Check sheet for the modelled part. Datum: model origin and axes. Units: mm. Coordinates: 2 decimals unless noted, no trailing zeros. Loops run counter-clockwise (first coordinate to the right, second up) from the corner with the lowest first, then second, coordinate; pieces in that order, holes last.
```python
from build123d import *

# Parameters (mm, degrees)
BOSS_EXTRUDE1_DEPTH = 2.5
FILLET1_R           = 3
FILLET2_R           = 3
FILLET4_R           = 3
FILLET5_R           = 3
SKETCH2_R           = 3
CUT_EXTRUDE1_DEPTH  = 3
FILLET6_R           = 3
FILLET7_R           = 3


with BuildPart() as part:
    # Sketch1 → Boss-Extrude1 (new body)
    with BuildSketch(Plane(origin=(0, 0, 0), x_dir=(1, 0, 0), z_dir=(0, 1, 0))):
        Polygon((-12.469879518, 24.84939759), (17.530120482, 24.84939759), (17.530120482, -5.15060241), (47.530120482, -5.15060241), (47.530120482, -35.15060241), (17.530120482, -35.15060241), (-12.469879518, -35.15060241), (-42.469879518, -35.15060241), (-42.469879518, -5.15060241), (-12.469879518, -5.15060241), align=None)
    extrude(amount=BOSS_EXTRUDE1_DEPTH)

    # Fillet1
    fillet1_edges = [part.edges().sort_by_distance(p)[0] for p in [
        (-42.469879518, 1.25, 5.15060241),
    ]]
    fillet(fillet1_edges, radius=FILLET1_R)

    # Fillet2
    fillet2_edges = [part.edges().sort_by_distance(p)[0] for p in [
        (-42.469879518, 1.25, 35.15060241),
    ]]
    fillet(fillet2_edges, radius=FILLET2_R)

    # Fillet4
    fillet4_edges = [part.edges().sort_by_distance(p)[0] for p in [
        (17.530120482, 1.25, -24.84939759),
    ]]
    fillet(fillet4_edges, radius=FILLET4_R)

    # Fillet5
    fillet5_edges = [part.edges().sort_by_distance(p)[0] for p in [
        (-12.469879518, 1.25, -24.84939759),
    ]]
    fillet(fillet5_edges, radius=FILLET5_R)

    # Sketch2 → Cut-Extrude1 (cut)
    with BuildSketch(Plane(origin=(0, 2.5, 0), x_dir=(1, 0, 0), z_dir=(0, 1, 0))):
        with Locations((2.530120482, 9.84939759)):
            Circle(SKETCH2_R)
        with Locations((-27.469879518, -20.15060241)):
            Circle(SKETCH2_R)
        with Locations((32.530120482, -20.15060241)):
            Circle(SKETCH2_R)
    extrude(amount=-CUT_EXTRUDE1_DEPTH, mode=Mode.SUBTRACT)

    # Fillet6
    fillet6_edges = [part.edges().sort_by_distance(p)[0] for p in [
        (47.530120482, 1.25, 35.15060241),
    ]]
    fillet(fillet6_edges, radius=FILLET6_R)

    # Fillet7
    fillet7_edges = [part.edges().sort_by_distance(p)[0] for p in [
        (47.530120482, 1.25, 5.15060241),
    ]]
    fillet(fillet7_edges, radius=FILLET7_R)


solid = part.part
```
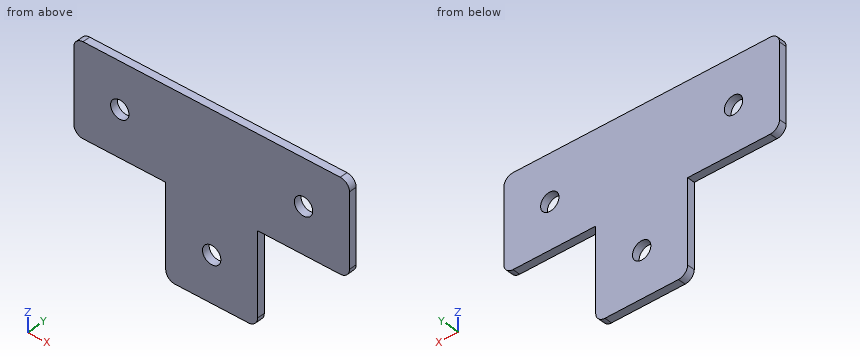
1) Section check D-D on z = -2. Enter the section's corners in (x, y), plus the area to 3 significant figures.
Answer sheet:
outline: (-12.47, 0) - (17.53, 0) - (17.53, 2.5) - (-12.47, 2.5) - close
area: 75.0 mm2
2) Section check C-C on y = 1.8. Enter the section's corners in (x, z).
Answer sheet:
outline: (-42.47, 8.15) arc R3 ccw to (-39.47, 5.15) - (-12.47, 5.15) - (-12.47, -21.85) arc R3 ccw to (-9.47, -24.85) - (14.53, -24.85) arc R3 ccw to (17.53, -21.85) - (17.53, 5.15) - (44.53, 5.15) arc R3 ccw to (47.53, 8.15) - (47.53, 32.15) arc R3 ccw to (44.53, 35.15) - (-39.47, 35.15) arc R3 ccw to (-42.47, 32.15) - close; hole circle Ø6 at (-27.47, 20.15); hole circle Ø6 at (2.53, -9.85); hole circle Ø6 at (32.53, 20.15)
3) Section check B-B on z = -8.5. Enter the section's corners in (x, y), plus the area to 3 significant figures.
Answer sheet:
outline: (-12.47, 0) - (-0.15, 0) - (-0.15, 2.5) - (-12.47, 2.5) - close; (5.21, 0) - (17.53, 0) - (17.53, 2.5) - (5.21, 2.5) - close
area: 61.6 mm2
4) Depth check by flat-ended pin: pin 1 (0.8 mm diameter, centred on y = 1, z = -9.5, fed in from +X); pin 2 (0.8 mm diameter, centred on y = 1.5, z = -2, fed in from -X). Enter the tip coordinate at first touch or a pass-through.
Answer sheet:
pin 1: stops at x = 17.53
pin 2: stops at x = -12.47
5) Section check A-A on x = -26. Enter the section's corners in (y, z), plus the area to 3 significant figures.
Answer sheet:
outline: (0, 5.15) - (2.5, 5.15) - (2.5, 17.54) - (0, 17.54) - close; (0, 22.77) - (2.5, 22.77) - (2.5, 35.15) - (0, 35.15) - close
area: 61.9 mm2
6) Scan lines: line 1 (Z direction, x = 32.5, y = 2.35); line 2 (Z direction, x = -33, y = 2.05); line 3 (X direction, y = 0.85, z = 0.5). Record each from-to range of solid material in increasing order.
Answer sheet:
line 1: z = 5.15 to 17.15, 23.15 to 35.15
line 2: z = 5.15 to 35.15
line 3: x = -12.47 to 17.53
